```python
from build123d import *

# Parameters (mm, degrees)
BOSS_EXTRUDE1_DEPTH            = 105
SKETCH2_R                      = 15
CUT_EXTRUDE1_DEPTH             = 1
CUT_EXTRUDE1_DEPTH_BACK        = 4.276608177
CUT_EXTRUDE2_REACH             = 5.277
SKETCH3_R                      = 2.5
CUT_EXTRUDE2_DIRECTION_2_DEPTH = 1
CUT_EXTRUDE3_REACH             = 5.277
SKETCH4_W                      = 13
SKETCH4_H                      = 19


with BuildPart() as part:
    # Sketch1 → Boss-Extrude1 (new body)
    with BuildSketch(Plane.XY):
        Polygon((-48.168421053, -4.926315789), (55.831578947, -4.926315789), (53.537273202, -1.649707612), (-45.874115307, -1.649707612), align=None)
    extrude(amount=-BOSS_EXTRUDE1_DEPTH)

    # Sketch2 → Cut-Extrude1 (cut, two sides)
    with BuildSketch(Plane(origin=(0, -1.649707612, 0), x_dir=(1, 0, 0), z_dir=(0, 1, 0))) as cut_extrude1_sk:
        with Locations((3.362524977, 35.234526985)):
            Circle(SKETCH2_R)
    extrude(amount=CUT_EXTRUDE1_DEPTH, mode=Mode.SUBTRACT)
    extrude(cut_extrude1_sk.sketch, amount=-CUT_EXTRUDE1_DEPTH_BACK, mode=Mode.SUBTRACT)

    # Sketch3 → Cut-Extrude2 (cut, up to next)
    with BuildSketch(Plane(origin=(0, -1.649707612, 0), x_dir=(1, 0, 0), z_dir=(0, 1, 0)), mode=Mode.PRIVATE) as cut_extrude2_sk1:
        with Locations((-36.016928445, 25.875156143)):
            Circle(SKETCH3_R)
    cut_extrude2_tool1 = extrude(cut_extrude2_sk1.sketch, amount=-CUT_EXTRUDE2_REACH, mode=Mode.PRIVATE) & part.part
    add(cut_extrude2_tool1.solids().sort_by_distance((-36.016928, -1.649708, -25.875156))[0], mode=Mode.SUBTRACT)
    # Sketch3 → Cut-Extrude2 (cut, up to next)
    with BuildSketch(Plane(origin=(0, -1.649707612, 0), x_dir=(1, 0, 0), z_dir=(0, 1, 0)), mode=Mode.PRIVATE) as cut_extrude2_sk2:
        with Locations((-36.016928445, 40.875156143)):
            Circle(SKETCH3_R)
    cut_extrude2_tool2 = extrude(cut_extrude2_sk2.sketch, amount=-CUT_EXTRUDE2_REACH, mode=Mode.PRIVATE) & part.part
    add(cut_extrude2_tool2.solids().sort_by_distance((-36.016928, -1.649708, -40.875156))[0], mode=Mode.SUBTRACT)

    # Sketch3 → Cut-Extrude2 direction 2 (cut)
    with BuildSketch(Plane(origin=(0, -1.649707612, 0), x_dir=(1, 0, 0), z_dir=(0, 1, 0))):
        with Locations((-36.016928445, 25.875156143)):
            Circle(SKETCH3_R)
        with Locations((-36.016928445, 40.875156143)):
            Circle(SKETCH3_R)
    extrude(amount=CUT_EXTRUDE2_DIRECTION_2_DEPTH, mode=Mode.SUBTRACT)

    # Sketch4 → Cut-Extrude3 (cut, up to next)
    with BuildSketch(Plane(origin=(0, -1.649707612, 0), x_dir=(1, 0, 0), z_dir=(0, 1, 0)), mode=Mode.PRIVATE) as cut_extrude3_sk1:
        with Locations((37.21482517, 36.119420448)):
            Rectangle(SKETCH4_W, SKETCH4_H)
    cut_extrude3_tool1 = extrude(cut_extrude3_sk1.sketch, amount=-CUT_EXTRUDE3_REACH, mode=Mode.PRIVATE) & part.part
    add(cut_extrude3_tool1.solids().sort_by_distance((37.214825, -1.649708, -36.11942))[0], mode=Mode.SUBTRACT)


solid = part.part
```
Can you work these out from the model? Positions are in its coordinate system, mm. A direction names the side the tool comes from. Round coordinates to 2 decimals unless told otherwise and drop trailing zeros. Loops run counter-clockwise (first coordinate to the right, second up) from the corner with the lowest first, then second, coordinate; pieces in that order, holes last.
Item 1: Will these pins go through, and if not, where does the flat tip stop? pin 1 Ø1.5 at (x, y) = (-30, -3.5) entering from +Z; pin 2 Ø1.5 at (y, z) = (-4, -48) entering from -X; pin 3 Ø1.6 at (y, z) = (-2.5, -35) entering from +X.
Item 2: Suppose I cut it at B-B, the plane y = -4.05. Write out the boundary of the cut face in (x, z), then the cut area to 3 significant figures.
Item 3: If we mould it in two halves opening along X, with no side actions, what happens to faces 3 (the flat face through (3, -4.926, -52)), 4 (the flat face through (54.7, -3.31, -51.76)), 5 (the flat face through (43.715, -3, -36))? For each: +X half, -X half, draft (parallel to the pull), parting line (faces both ways), or undercut.
Item 4: Please list where these lines run through material, in increasing order: L1, parallel to X at y = -3.8, z = -30.5; L2, parallel to X at y = -3.1, z = -44; L3, parallel to X at y = -1.9, z = -40.
Item 5: Suppose I cut it at D-D, the plane x = -36. Write out the boundary of the cut face in (y, z), then the cut area to 3 significant figures.
Item 6: Which directions (+Z, -Z, +X, -X, +Y, -Y) give clear straight access to the entire face, cutting with the end or side of a thin tool? Please do faces 1 (the flat face through (3, -3, -105)), 2 (the flat face through (37, -3, -45.619)).
Item 7: Suppose I cut it at C-C, the plane z = -89. Write out the boundary of the cut face in (x, y), then the cut area to 3 significant figures.
Item 8: Suppose I cut it at A-A, the plane x = 41.5. Write out the boundary of the cut face in (y, z).
Reported:
1. pin 1: stops at z = 0
1. pin 2: stops at x = -48.04
1. pin 3: stops at x = 54.69
2. outline: (-47.55, -105) - (55.22, -105) - (55.22, 0) - (-47.55, 0) - close; hole circle Ø5 at (-36.02, -40.88); hole circle Ø5 at (-36.02, -25.88); hole circle Ø30 at (3.36, -35.23); hole (30.71, -45.62) - (43.71, -45.62) - (43.71, -26.62) - (30.71, -26.62) - close
2. area: 9,800 mm2
3. face 3: draft
3. face 4: +X half
3. face 5: undercut
4. L1: x = -47.38 to -10.87, 17.6 to 30.71, 43.71 to 55.04
4. L2: x = -46.89 to -8.81, 15.53 to 30.71, 43.71 to 54.55
4. L3: x = -46.05 to -38.36, -33.68 to -10.86, 17.59 to 30.71, 43.71 to 53.71
5. outline: (-4.93, -105) - (-1.65, -105) - (-1.65, -43.38) - (-4.93, -43.38) - close; (-4.93, -38.38) - (-1.65, -38.38) - (-1.65, -28.38) - (-4.93, -28.38) - close; (-4.93, -23.38) - (-1.65, -23.38) - (-1.65, 0) - (-4.93, 0) - close
5. area: 311 mm2
6. face 1: -Z, +X, -X, +Y, -Y
6. face 2: +Y, -Y
7. outline: (-48.17, -4.93) - (55.83, -4.93) - (53.54, -1.65) - (-45.87, -1.65) - close
7. area: 333 mm2
8. outline: (-4.93, -105) - (-1.65, -105) - (-1.65, -45.62) - (-4.93, -45.62) - close; (-4.93, -26.62) - (-1.65, -26.62) - (-1.65, 0) - (-4.93, 0) - close
